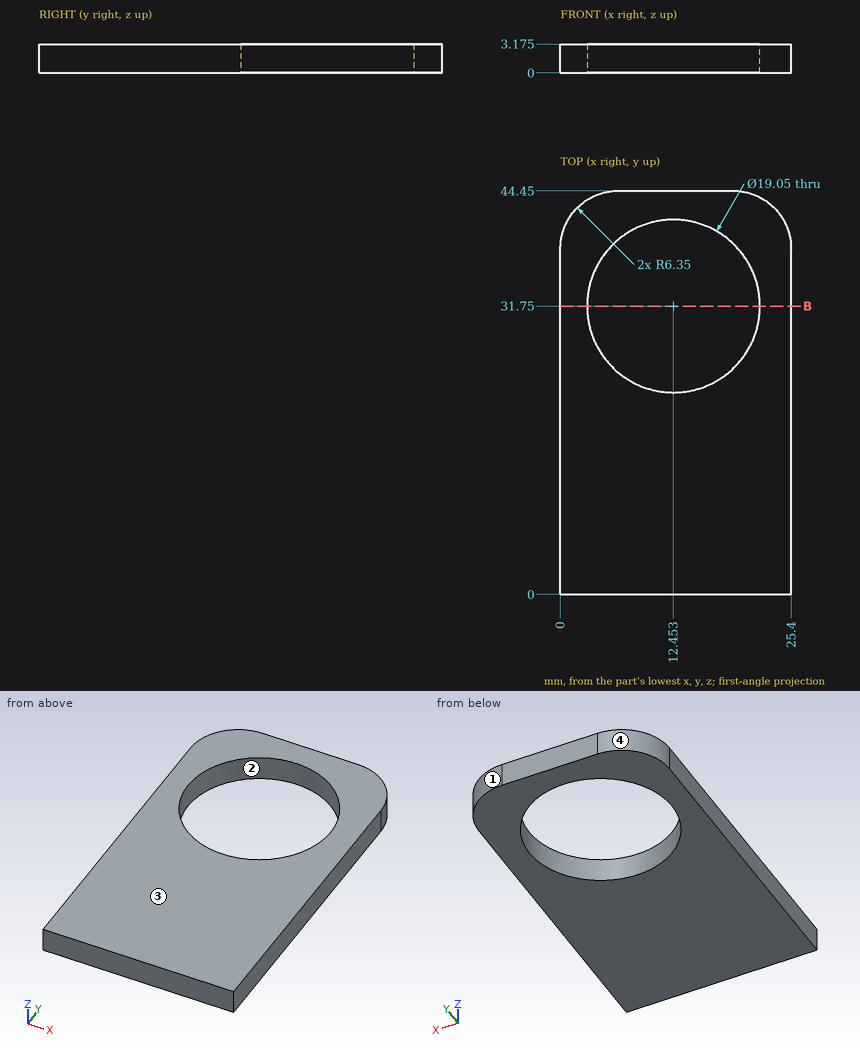
Drawing for the job (mm, zero at the part's lowest x, y, z). Round coordinates to 2 decimals unless told otherwise and drop trailing zeros. Loops run counter-clockwise (first coordinate to the right, second up) from the corner with the lowest first, then second, coordinate; pieces in that order, holes last.
1. Wall check: probe 1 along Y at (x, z) = (12.75, 2.7); probe 2 along X at (y, z) = (31.5, 2.95) (1 decimal); probe 3 along X at (y, z) = (28, 2.2). Give the ranges that are in metal, low to high.
Check values:
probe 1: y = 0 to 22.23, 41.27 to 44.45
probe 2: x = 0 to 2.9, 22 to 25.4
probe 3: x = 0 to 3.7, 21.21 to 25.4
2. Band-saw the part on B-B, the plane y = 31.75. List the corners of the cut face in (x, z) (1 decimal).
Check values:
outline: (0, 0) - (2.9, 0) - (2.9, 3.2) - (0, 3.2) - close; (22, 0) - (25.4, 0) - (25.4, 3.2) - (22, 3.2) - close
3. Drop flat-ended pins along their axis: P1, Ø1, axis at x = 4.5, z = 2, coming from the +Y side (1 decimal); P2, Ø10, axis at x = 17, y = 33, coming from the -Z side. Give the stop position or say it passes through.
Check values:
P1: stops at y = 44.3
P2: stops at z = 0
4. Mould opens along X. For the marked faces 1, 2, 3 and 4 say: +X half, -X half, draft (parallel to the pull), parting line (faces both ways), or undercut.
Check values:
face 1: +X half
face 2: undercut
face 3: draft
face 4: -X half
